from build123d import *

# Parameters (mm, degrees)
BOSS_EXTRUDE1_DEPTH = 81.28
SHELL2_T            = -1.27
BOSS_EXTRUDE2_DEPTH = 81.28


with BuildPart() as part:
    # Sketch1 → Boss-Extrude1 (new body)
    with BuildSketch(Plane.XY):
        with BuildLine():
            Line((-31.75, 0), (31.75, 0))
            ThreePointArc((31.75, 0), (0, 31.75), (-31.75, 0))
        make_face()
    extrude(amount=-BOSS_EXTRUDE1_DEPTH)

    # Shell2
    shell2_openings = [part.faces().sort_by_distance(p)[0] for p in [
        (0, 13.475118515, 0),
    ]]
    offset(amount=SHELL2_T, openings=shell2_openings)

    # Sketch5 → Boss-Extrude2 (add)
    with BuildSketch(Plane.XY):
        with BuildLine():
            Line((-3.8e-08, 0), (-31.75, 0))
            Line((-31.75, 0), (-31.75, -25.527))
            Line((-31.75, -25.527), (-25.527, -25.527))
            ThreePointArc((-25.527, -25.527), (-18.050314817, -7.47668521), (-3.8e-08, 0))
        make_face()
        with BuildLine():
            Line((31.75, 0), (-3.8e-08, 0))
            ThreePointArc((-3.8e-08, 0), (18.05031479, -7.476685183), (25.527, -25.527))
            Line((25.527, -25.527), (31.75, -25.527))
            Line((31.75, -25.527), (31.75, 0))
        make_face()
    extrude(amount=-BOSS_EXTRUDE2_DEPTH)


solid = part.part
Could you check a few things on this model? Use its own coordinates, in mm. A direction names the side the tool comes from. Give positions to 0.01 mm unless a question says otherwise; leave off trailing zeros. Order: outer loops, then holes, each group sorted by start corner. A loop starts at its lowest first (then second) coordinate and runs counter-clockwise, first axis right, second up. Notation, with made-up numbers: (-8, 63.25) -> (17, 63.25) arc R18 cw to (17, 96.25) -> close; hole circle Ø10 at (66, 89). An arc over 180 degrees is marked (long way). Return JSON: item names as keys, results as strings.
1. Imagine slicing it at B-B on y = -9. List the corners of the cut face in (x, z) for me.
Answer list:
{"outline": "(-31.75, -81.28) -> (-19.45, -81.28) -> (-19.45, 0) -> (-31.75, 0) -> close; (19.45, -81.28) -> (31.75, -81.28) -> (31.75, 0) -> (19.45, 0) -> close"}
2. Imagine slicing it at A-A on z = -65. List the corners of the cut face in (x, y) for me, then the cut area to 3 significant figures.
Answer list:
{"outline": "(-31.75, -25.53) -> (-25.53, -25.53) arc R25.53 cw to (25.53, -25.53) -> (31.75, -25.53) -> (31.75, 0) arc R31.75 ccw to (-31.75, 0) -> close; hole (-30.45, 1.27) -> (30.45, 1.27) arc R30.48 ccw to start", "area": "799 mm2"}
3. For pin 1 Ø4 at (x, z) = (-13.5, -37.5) entering from -Y; pin 2 Ø8 at (y, z) = (23.5, -64.5) entering from -X; pin 3 Ø2 at (x, y) = (8, 21.5) entering from +Z, each with a flat end and sliding along its axis, tell me the tip position at first contact or that it passes through.
Answer list:
{"pin 1": "stops at y = -5.24", "pin 2": "stops at x = -25.06", "pin 3": "stops at z = -80.01"}
4. On a 3-axis mill with a long thin cutter (end or side, diameter ignored), from which of +Z, -Z, +X, -X, +Y, -Y can I reach the whole of each face in a straight line? I mean faces 1 (the cylindrical face through (0.652, 30.473, -39.445)), 2 (the flat face through (29, -25.527, -40)). Say none if no direction works.
Answer list:
{"face 1": "+Z", "face 2": "+Z, -Z, +X, -X, -Y"}
5. Thinking about a two-plate mould opening in Y: for faces 3 (the flat face through (-31.75, -13, -40)), 4 (the flat face through (-29, -25.527, -40)), 5 (the flat face through (0, 1.27, -39)), 6 (the flat face through (0, 13, -80.01)), which applies, pulls with the +Y half, pulls with the -Y half, needs draft (parallel to the pull), parting line crosses it, or undercut?
Answer list:
{"face 3": "needs draft", "face 4": "pulls with the -Y half", "face 5": "undercut", "face 6": "undercut"}
6. Imagine slicing it at D-D on y = 27.5. List the corners of the cut face in (x, z) for me, then the cut area to 3 significant figures.
Answer list:
{"outline": "(-15.87, -81.28) -> (15.87, -81.28) -> (15.87, 0) -> (13.14, 0) -> (13.14, -80.01) -> (-13.14, -80.01) -> (-13.14, 0) -> (-15.87, 0) -> close", "area": "476 mm2"}
7. I need wall thicknesses on line 1 (Y direction, x = 0.5, z = -70); line 2 (Y direction, x = -15, z = -60.5); line 3 (X direction, y = 18, z = -37). Which ranges of each line are inside material? Lowest first, please. Write a range as from..to.
Answer list:
{"line 1": "y = 0..1.27, 30.48..31.75", "line 2": "y = -4.87..1.27, 26.53..27.98", "line 3": "x = -26.15..-24.6, 24.6..26.15"}
8. Imagine slicing it at C-C on x = -11. List the corners of the cut face in (y, z) for me, then the cut area to 3 significant figures.
Answer list:
{"outline": "(-2.49, -81.28) -> (29.78, -81.28) -> (29.78, 0) -> (28.43, 0) -> (28.43, -80.01) -> (1.27, -80.01) -> (1.27, 0) -> (-2.49, 0) -> close", "area": "451 mm2"}
